```python
from build123d import *

# Parameters (mm, degrees)
SKETCH1_W           = 20.480821918
SKETCH1_H           = 31.9
SKETCH1_R           = 2.45
BOSS_EXTRUDE1_DEPTH = 4
SKETCH2_W           = 18.980821918
SKETCH2_H           = 9.35
CUT_EXTRUDE1_DEPTH  = 3
SKETCH3_R           = 1.5
BOSS_EXTRUDE2_DEPTH = 8
SKETCH4_W           = 18.980821918
SKETCH4_H           = 1.5
BOSS_EXTRUDE3_DEPTH = 1.3
SKETCH5_W           = 5.480821918
SKETCH5_H           = 31.9
CUT_EXTRUDE2_DEPTH  = 7.4
SKETCH6_W           = 6
SKETCH6_H           = 4
CUT_EXTRUDE3_DEPTH  = 4
FILLET1_R           = 3
FILLET2_R           = 1
FILLET3_R           = 0.5
SKETCH7_R           = 3.25
CUT_EXTRUDE4_DEPTH  = 1


with BuildPart() as part:
    # Sketch1 → Boss-Extrude1 (new body)
    with BuildSketch(Plane.XY):
        Rectangle(SKETCH1_W, SKETCH1_H)
        with Locations((6.290410959, 12)):
            Circle(SKETCH1_R, mode=Mode.SUBTRACT)
        with Locations((6.290410959, -12)):
            Circle(SKETCH1_R, mode=Mode.SUBTRACT)
    extrude(amount=BOSS_EXTRUDE1_DEPTH)

    # Sketch2 → Cut-Extrude1 (cut)
    with BuildSketch(Plane.XY.offset(4)):
        with Locations((-0.75, 4.675)):
            Rectangle(SKETCH2_W, SKETCH2_H)
        with Locations((-0.75, -4.675)):
            Rectangle(SKETCH2_W, SKETCH2_H)
    extrude(amount=-CUT_EXTRUDE1_DEPTH, mode=Mode.SUBTRACT)

    # Sketch3 → Boss-Extrude2 (add)
    with BuildSketch(Plane.XY.offset(1)):
        with Locations((-1.259589041, 5)):
            Circle(SKETCH3_R)
        with Locations((-1.259589041, -5)):
            Circle(SKETCH3_R)
    extrude(amount=BOSS_EXTRUDE2_DEPTH)

    # Sketch4 → Boss-Extrude3 (add)
    with BuildSketch(Plane.XY.offset(1)):
        with Locations((-0.75, 8.6)):
            Rectangle(SKETCH4_W, SKETCH4_H)
        with Locations((-0.75, -8.6)):
            Rectangle(SKETCH4_W, SKETCH4_H)
    extrude(amount=BOSS_EXTRUDE3_DEPTH)

    # Sketch5 → Cut-Extrude2 (cut)
    with BuildSketch(Plane.XY.offset(4)):
        with Locations((-7.5, 0)):
            Rectangle(SKETCH5_W, SKETCH5_H)
    extrude(amount=-CUT_EXTRUDE2_DEPTH, mode=Mode.SUBTRACT)

    # Sketch6 → Cut-Extrude3 (cut)
    with BuildSketch(Plane.XY.offset(4)):
        with Locations((-1.759589041, 13.95)):
            Rectangle(SKETCH6_W, SKETCH6_H)
        with Locations((-1.759589041, -13.95)):
            Rectangle(SKETCH6_W, SKETCH6_H)
    extrude(amount=-CUT_EXTRUDE3_DEPTH, mode=Mode.SUBTRACT)

    # Fillet1
    fillet1_edges = [part.edges().sort_by_distance(p)[0] for p in [
        (10.240410959, 15.95, 2),
        (10.240410959, -15.95, 2),
        (1.240410959, -15.95, 2),
        (-4.759589041, -11.95, 2),
        (-4.759589041, 11.95, 2),
        (1.240410959, 15.95, 2),
    ]]
    fillet(fillet1_edges, radius=FILLET1_R)

    # Fillet2
    fillet2_edges = [part.edges().sort_by_distance(p)[0] for p in [
        (-2.759589041, 5, 1),
        (-2.759589041, -5, 1),
    ]]
    fillet(fillet2_edges, radius=FILLET2_R)

    # Fillet3
    fillet3_edges = [part.edges().sort_by_distance(p)[0] for p in [
        (-2.759589041, 5, 9),
        (-2.759589041, -5, 9),
    ]]
    fillet(fillet3_edges, radius=FILLET3_R)

    # Sketch7 → Cut-Extrude4 (cut)
    with BuildSketch(Plane(origin=(0, 0, 0), x_dir=(-1, 0, 0), z_dir=(0, 0, -1))):
        with Locations((-6.290410959, 12)):
            Circle(SKETCH7_R)
        with Locations((-6.290410959, -12)):
            Circle(SKETCH7_R)
    extrude(amount=-CUT_EXTRUDE4_DEPTH, mode=Mode.SUBTRACT)


solid = part.part
```
The model under review builds one solid part; all positions refer to its coordinate system, in mm. A direction names the side the tool comes from. Round coordinates to 2 decimals unless told otherwise and drop trailing zeros. Loops run counter-clockwise (first coordinate to the right, second up) from the corner with the lowest first, then second, coordinate; pieces in that order, holes last. Notation, with made-up numbers: M -14,-16.5 L 16,-16.5 A28 cw 16,10.5 Z; hole C 47.25,-28 d8. An arc over 180 degrees is marked long. Put each result on its own line as item: value.
Q1. Consider section D-D, the plane y = -0.5. Give the boundary of the cut face in (x, z).
Result set:
outline: M -4.76,0 L 10.24,0 L 10.24,4 L 8.74,4 L 8.74,1 L -4.76,1 Z
Q2. Mouldability with a two-part tool opening along X and no side actions: class faces 1 (the flat face through (1.24, 12.4, 2)), 2 (the flat face through (2, -7.85, 2)), 3 (the cylindrical face through (3.2, 13, 0.5)) as released by +X, released by -X, zero draft, split by the parting line, or undercut.
Result set:
face 1: released by -X
face 2: zero draft
face 3: undercut
Q3. For pin 1 (1.2 mm diameter, centred on x = 2.5, y = -8.5, fed in from +Z); pin 2 (3.5 mm diameter, centred on x = 0, z = 1.5, fed in from -Y); pin 3 (5 mm diameter, centred on x = 6.29, y = -12, fed in from -Z), all flat-tipped, find the tip position at first contact; note any pin that passes through.
Result set:
pin 1: stops at z = 2.3
pin 2: stops at y = -14.62
pin 3: stops at z = 1
Q4. To check wall thickness, follow L1, parallel to X at y = -12, z = 2; L2, parallel to Y at x = 7.25, z = 2; L3, parallel to Y at x = 8, z = 3.75. State the ranges of each line that lie inside material, in increasing order.
Result set:
L1: x = 1.24 to 3.84, 8.74 to 10.24
L2: y = -15.95 to -14.25, -9.75 to -7.85, 7.85 to 9.75, 14.25 to 15.95
L3: y = -15.85 to -13.75, -10.25 to -9.35, 9.35 to 10.25, 13.75 to 15.85
Q5. Consider section B-B, the plane z = 5.75. Give the boundary of the cut face in (x, y).
Result set:
outline: C -1.26,-5 d3; C -1.26,5 d3
Q6. Consider section A-A, the plane x = 6.75. Give the boundary of the cut face in (y, z), then the cut area to 3 significant figures.
Result set:
outline: M -15.95,0 L -15.22,0 L -15.22,1 L -14.41,1 L -14.41,4 L -15.95,4 Z; M -9.59,1 L -8.78,1 L -8.78,0 L 8.78,0 L 8.78,1 L 9.59,1 L 9.59,4 L 9.35,4 L 9.35,2.3 L 7.85,2.3 L 7.85,1 L -7.85,1 L -7.85,2.3 L -9.35,2.3 L -9.35,4 L -9.59,4 Z; M 14.41,1 L 15.22,1 L 15.22,0 L 15.95,0 L 15.95,4 L 14.41,4 Z
area: 33.7 mm²
Q7. Consider section C-C, the plane y = -5. Give the boundary of the cut face in (x, z), then the cut area to 3 significant figures.
Result set:
outline: M -4.76,0 L 10.24,0 L 10.24,4 L 8.74,4 L 8.74,1 L 1.24,1 A1 cw 0.24,2 L 0.24,8.5 A0.5 ccw -0.26,9 L -2.26,9 A0.5 ccw -2.76,8.5 L -2.76,2 A1 cw -3.76,1 L -4.76,1 Z
area: 43.8 mm²
Q8. Machinability: for faces 4 (the flat face through (3, 0, 1)), 5 (the flat face through (2, 9.35, 3)), 6 (the flat face through (6, -15.95, 2)), 7 (the flat face through (8, -10, 1)), 8 (the flat face through (0, -11.95, 2)), which of the approach directions +Z, -Z, +X, -X, +Y, -Y give a long, thin tool a straight path to every point of the face, cutting with its end or side? Answer none if there is none.
Result set:
face 4: +Z
face 5: +Z, -X
face 6: +Z, -Z, +X, -X, -Y
face 7: -Z
face 8: +Z, -Z, -X, -Y
